Input: part model. Units: mm. Frame: model coordinates. A direction names the side the tool comes from. Give positions to 0.01 mm unless a question says otherwise; leave off trailing zeros. Loops run counter-clockwise (first coordinate to the right, second up) from the corner with the lowest first, then second, coordinate; pieces in that order, holes last. Notation, with made-up numbers: M -25,-8.75 L 4,-8.75 A18 ccw 4,-1.75 Z; hole C -35,69.5 d10. An arc over 180 degrees is marked long. Return JSON: item names as keys, results as strings. Group by question number.
```python
from build123d import *

# Parameters (mm, degrees)
F0_W     = 80.6774497032
F0_H     = 79.8543840647
F1_DEPTH = 50
F2_SIZE2 = 9.99999
F2_SIZE  = 49.99999
F3_R     = 2.5976453029
F4_DEPTH = 15


# Not quite as in the source:
# - a fillet or chamfer is up to 0.001 mm smaller than in the source, because OpenCascade refuses the exact size


with BuildPart() as f1:
    # F0 (on Top) → F1 (new body)
    with BuildSketch(Plane.XY):
        with Locations((0.1392643899, 1.1030137539)):
            Rectangle(F0_W, F0_H)
    extrude(amount=-F1_DEPTH)

    # F2 (size 50 and 10 in the source; OpenCascade refuses exactly that, so slightly less here)
    f2_edges = [f1.edges().sort_by_distance(p)[0] for p in [
        (0.139264, 41.030206, 0),
        (-40.19946, 1.103014, 0),
        (0.139264, -38.824178, 0),
        (40.477989, 1.103014, 0),
    ]]
    chamfer(f2_edges, length=F2_SIZE, length2=F2_SIZE2)

    # F3 (on Top) → F4 (join)
    with BuildSketch(Plane.XY):
        Circle(F3_R)
    extrude(amount=F4_DEPTH)


solid = f1.part
```
Item 1: Material intervals for line 1 (Z direction, x = -18, y = -6.5); line 2 (X direction, y = 32.5, z = -27); line 3 (X direction, y = -3.5, z = -22), sorted ascending. Write a range as from..to.
Item 2: Section C-C, the plane z = -16. Return loops of the section in (x, y).
Item 3: Reachability of faces 1 (the face through (35.4, 0.5, -24.6)), 2 (the face through (-0.563, -2.536, 7.395)) from +Z, -Z, +X, -X, +Y, -Y: full face, straight path, thin tool, end or side. Return the list, or none.
Item 4: First-contact query: pin 1 Ø6 at (x, y) = (9, -6.5) entering from +Z; pin 2 Ø5 at (x, z) = (-9, -23) entering from -Y; pin 3 Ø12 at (x, z) = (-8, 4.5) entering from +Y. Flat tips, straight axial feed; report the tip coordinate or a pass-through.
Answer below:
{
 "1": {"line 1": "-50..0", "line 2": "-35.6..35.88", "line 3": "-34.6..34.88"},
 "2": {"outline": "M -33.4,-32.02 L 33.68,-32.02 L 33.68,34.23 L -33.4,34.23 Z"},
 "3": {"face 1": "+Z, +X, +Y, -Y", "face 2": "+Z"},
 "4": {"pin 1": "z = 0", "pin 2": "y = -33.92", "pin 3": "y = 31.33"}
}
